Read the model definition and answer for the solid it produces. Units are mm, in the model's axes. Coordinates: 2 decimals unless noted, no trailing zeros. Write each loop counter-clockwise with the first axis right and the second up, starting at its lowest first coordinate (ties: lowest second). Pieces come first, ordered by that corner, then holes. Notation, with made-up numbers: (78.25, 86.5) -> (118.25, 86.5) arc R7 cw to (118.25, 96.5) -> close; hole circle Ø2 at (-7, 48). An arc over 180 degrees is marked (long way). One line per item, written item: value. Start each with the question number.
1. Given P1, Ø8, axis at y = 277.5, z = -418.5, coming from the -X side; P2, Ø1.5, axis at y = 273, z = -426, coming from the +X side; P3, Ø1, axis at x = 1, z = -392, coming from the -Y side, each flat-ended and moving along its own axis, determine where each tip first touches the part or whether it passes through.
2. Consider line 1 along Y through (x, z) = (0.6, -349); line 2 along Z through (x, y) = (2.7, 335.5); line 3 along Y through (x, z) = (2.2, -310). Determine where each line is inside the solid, lowest interval first.
3. Find section A-A, the plane z = -381. Write down the section's boundary in (x, y) (3 decimals).
4. Find section B-B, the plane y = 323.85. State how many separate pieces and enclosed holes the cut face has, and give its area (3 significant figures).
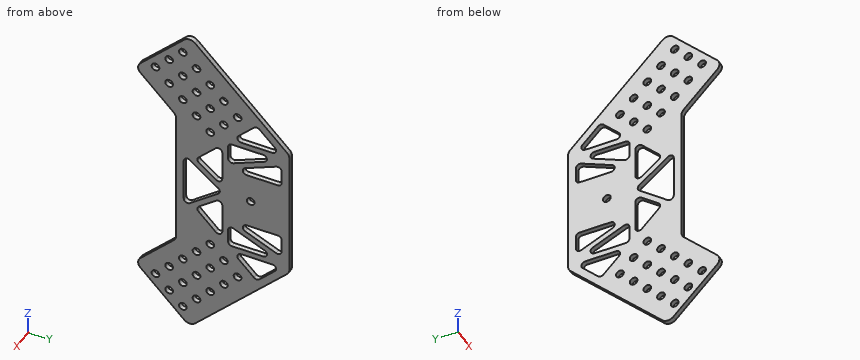
```python
from build123d import *

# Parameters (mm, degrees)
SKETCH7_R           = 2.54
BOSS_EXTRUDE1_DEPTH = 3.175
FILLET1_R           = 2.54
FILLET2_R           = 5.08


with BuildPart() as part:
    # Sketch7 → Boss-Extrude1 (new body)
    with BuildSketch(Plane(origin=(0, 0, 0), x_dir=(0, 0, -1), z_dir=(1, 0, 0))):
        Polygon((307.056403027, 247.914354058), (333.99717139, 274.855122421), (428.00282861, 274.855122421), (454.943596973, 247.914354058), (490.864621458, 283.835378542), (425.45, 349.25), (336.55, 349.25), (271.135378542, 283.835378542), align=None)
        with Locations((284.605762724, 279.345250482)):
            Circle(SKETCH7_R, mode=Mode.SUBTRACT)
        with Locations((293.586018845, 288.325506603)):
            Circle(SKETCH7_R, mode=Mode.SUBTRACT)
        with Locations((302.566274966, 297.305762724)):
            Circle(SKETCH7_R, mode=Mode.SUBTRACT)
        with Locations((311.546531087, 306.286018845)):
            Circle(SKETCH7_R, mode=Mode.SUBTRACT)
        with Locations((320.526787208, 315.266274966)):
            Circle(SKETCH7_R, mode=Mode.SUBTRACT)
        with Locations((302.566274966, 279.345250482)):
            Circle(SKETCH7_R, mode=Mode.SUBTRACT)
        with Locations((311.546531087, 288.325506603)):
            Circle(SKETCH7_R, mode=Mode.SUBTRACT)
        with Locations((320.526787208, 297.305762724)):
            Circle(SKETCH7_R, mode=Mode.SUBTRACT)
        with Locations((329.507043329, 306.286018845)):
            Circle(SKETCH7_R, mode=Mode.SUBTRACT)
        with Locations((311.546531087, 270.364994361)):
            Circle(SKETCH7_R, mode=Mode.SUBTRACT)
        with Locations((320.526787208, 279.345250482)):
            Circle(SKETCH7_R, mode=Mode.SUBTRACT)
        with Locations((329.507043329, 288.325506603)):
            Circle(SKETCH7_R, mode=Mode.SUBTRACT)
        with Locations((338.48729945, 297.305762724)):
            Circle(SKETCH7_R, mode=Mode.SUBTRACT)
        with Locations((293.586018845, 270.364994361)):
            Circle(SKETCH7_R, mode=Mode.SUBTRACT)
        with Locations((302.566274966, 261.38473824)):
            Circle(SKETCH7_R, mode=Mode.SUBTRACT)
        with Locations((477.394237276, 279.345250482)):
            Circle(SKETCH7_R, mode=Mode.SUBTRACT)
        with Locations((468.413981155, 288.325506603)):
            Circle(SKETCH7_R, mode=Mode.SUBTRACT)
        with Locations((459.433725034, 297.305762724)):
            Circle(SKETCH7_R, mode=Mode.SUBTRACT)
        with Locations((450.453468913, 306.286018845)):
            Circle(SKETCH7_R, mode=Mode.SUBTRACT)
        with Locations((441.473212792, 315.266274966)):
            Circle(SKETCH7_R, mode=Mode.SUBTRACT)
        with Locations((459.433725034, 279.345250482)):
            Circle(SKETCH7_R, mode=Mode.SUBTRACT)
        with Locations((450.453468913, 288.325506603)):
            Circle(SKETCH7_R, mode=Mode.SUBTRACT)
        with Locations((441.473212792, 297.305762724)):
            Circle(SKETCH7_R, mode=Mode.SUBTRACT)
        with Locations((432.492956671, 306.286018845)):
            Circle(SKETCH7_R, mode=Mode.SUBTRACT)
        with Locations((450.453468913, 270.364994361)):
            Circle(SKETCH7_R, mode=Mode.SUBTRACT)
        with Locations((441.473212792, 279.345250482)):
            Circle(SKETCH7_R, mode=Mode.SUBTRACT)
        with Locations((432.492956671, 288.325506603)):
            Circle(SKETCH7_R, mode=Mode.SUBTRACT)
        with Locations((423.51270055, 297.305762724)):
            Circle(SKETCH7_R, mode=Mode.SUBTRACT)
        with Locations((468.413981155, 270.364994361)):
            Circle(SKETCH7_R, mode=Mode.SUBTRACT)
        with Locations((459.433725034, 261.38473824)):
            Circle(SKETCH7_R, mode=Mode.SUBTRACT)
        with Locations((381, 323.85)):
            Circle(SKETCH7_R, mode=Mode.SUBTRACT)
        Polygon((322.322838433, 327.838633536), (338.654204897, 344.17), (338.654204897, 311.507267071), align=None, mode=Mode.SUBTRACT)
        Polygon((342.464204897, 344.17), (342.464204897, 309.023397149), (357.793385063, 309.023397149), align=None, mode=Mode.SUBTRACT)
        Polygon((346.620819834, 344.17), (361.95, 344.17), (361.95, 309.023397149), align=None, mode=Mode.SUBTRACT)
        Polygon((344.94807482, 305.213397149), (362.606349547, 287.555122421), (376.192769102, 305.213397149), align=None, mode=Mode.SUBTRACT)
        Polygon((400.449309255, 279.935122421), (361.550690745, 279.935122421), (381, 305.213397149), align=None, mode=Mode.SUBTRACT)
        Polygon((400.05, 309.023397149), (400.05, 344.17), (415.379180166, 344.17), align=None, mode=Mode.SUBTRACT)
        Polygon((385.807230898, 305.213397149), (417.05192518, 305.213397149), (399.393650453, 287.555122421), align=None, mode=Mode.SUBTRACT)
        Polygon((404.206614937, 309.023397149), (419.535795103, 344.17), (419.535795103, 309.023397149), align=None, mode=Mode.SUBTRACT)
        Polygon((423.345795103, 311.507267071), (439.677161567, 327.838633536), (423.345795103, 344.17), align=None, mode=Mode.SUBTRACT)
    extrude(amount=BOSS_EXTRUDE1_DEPTH)

    # Fillet1
    fillet1_edges = [part.edges().sort_by_distance(p)[0] for p in [
        (1.5875, 309.023397149, -404.206614937),
        (1.5875, 309.023397149, -419.535795103),
        (1.5875, 344.17, -419.535795103),
        (1.5875, 305.213397149, -385.807230898),
        (1.5875, 287.555122421, -399.393650453),
        (1.5875, 305.213397149, -417.05192518),
        (1.5875, 344.17, -338.654204897),
        (1.5875, 327.838633536, -322.322838433),
        (1.5875, 311.507267071, -338.654204897),
        (1.5875, 344.17, -342.464204897),
        (1.5875, 309.023397149, -342.464204897),
        (1.5875, 309.023397149, -357.793385063),
        (1.5875, 305.213397149, -344.94807482),
        (1.5875, 287.555122421, -362.606349547),
        (1.5875, 305.213397149, -376.192769102),
        (1.5875, 344.17, -361.95),
        (1.5875, 344.17, -346.620819834),
        (1.5875, 309.023397149, -361.95),
        (1.5875, 305.213397149, -381),
        (1.5875, 279.935122421, -361.550690745),
        (1.5875, 279.935122421, -400.449309255),
        (1.5875, 344.17, -400.05),
        (1.5875, 309.023397149, -400.05),
        (1.5875, 344.17, -415.379180166),
        (1.5875, 344.17, -423.345795103),
        (1.5875, 311.507267071, -423.345795103),
        (1.5875, 327.838633536, -439.677161567),
    ]]
    fillet(fillet1_edges, radius=FILLET1_R)

    # Fillet2
    fillet2_edges = [part.edges().sort_by_distance(p)[0] for p in [
        (1.5875, 349.25, -425.45),
        (1.5875, 283.835378542, -490.864621458),
        (1.5875, 247.914354058, -454.943596973),
        (1.5875, 274.855122421, -428.00282861),
        (1.5875, 274.855122421, -333.99717139),
        (1.5875, 247.914354058, -307.056403027),
        (1.5875, 283.835378542, -271.135378542),
        (1.5875, 349.25, -336.55),
    ]]
    fillet(fillet2_edges, radius=FILLET2_R)


solid = part.part
```
Answer block:
1. P1: stops at x = 0
1. P2: passes through
1. P3: stops at y = 274.86
2. line 1: y = 274.86 to 301.22, 304.13 to 309.02, 329.18 to 338.72, 343.68 to 349.25
2. line 2: z = -439.2 to -432.02, -423.35 to -411.6, -400.05 to -361.95, -350.4 to -338.65, -329.98 to -322.8
2. line 3: y = 250.96 to 268.35, 272.38 to 286.31, 290.34 to 304.27, 308.3 to 322.7
3. outline: (0, 274.855) -> (3.175, 274.855) -> (3.175, 279.935) -> (0, 279.935) -> close; (0, 303.588) -> (3.175, 303.588) -> (3.175, 321.31) -> (0, 321.31) -> close; (0, 326.39) -> (3.175, 326.39) -> (3.175, 349.25) -> (0, 349.25) -> close
4. separate pieces: 8
4. enclosed holes: 0
4. area: 252 mm2
